```python
from build123d import *

# Parameters (mm, degrees)
SKETCH1_W           = 20
SKETCH1_H           = 16
BOSS_EXTRUDE1_DEPTH = 1.5
BOSS_EXTRUDE2_DEPTH = 2.6
CUT_EXTRUDE1_DEPTH  = 1
SKETCH4_R           = 1.85
CUT_EXTRUDE2_DEPTH  = 1.3
CUT_EXTRUDE3_DEPTH  = 4.3
FILLET1_R           = 1


with BuildPart() as part:
    # Sketch1 → Boss-Extrude1 (new body)
    with BuildSketch(Plane(origin=(0, 0, 0), x_dir=(1, 0, 0), z_dir=(0, 1, 0))):
        Rectangle(SKETCH1_W, SKETCH1_H)
    extrude(amount=BOSS_EXTRUDE1_DEPTH)

    # Sketch2 → Boss-Extrude2 (add)
    with BuildSketch(Plane.ZY.offset(10)):
        with BuildLine():
            Line((8, 0), (8, 5))
            Line((8, 5), (-5.076696831, 10))
            Line((-5.076696831, 10), (-13, 10))
            Line((-13, 10), (-13.5, 8.25))
            Line((-13.5, 8.25), (-16.8, 8.25))
            ThreePointArc((-16.8, 8.25), (-18.4, 5), (-16.8, 1.75))
            Line((-16.8, 1.75), (-13.5, 1.75))
            Line((-13.5, 1.75), (-13, 0))
            Line((-13, 0), (8, 0))
        make_face()
    boss_extrude2 = extrude(amount=-BOSS_EXTRUDE2_DEPTH)

    # Sketch3 → Cut-Extrude1 (cut)
    with BuildSketch(Plane(origin=(-7.4, 0, 0), x_dir=(0, 0, -1), z_dir=(1, 0, 0))):
        Polygon((-8, 1.5), (4.4, 1.5), (4.4, 9.7412585), (-8, 5), align=None)
    cut_extrude1 = extrude(amount=-CUT_EXTRUDE1_DEPTH, mode=Mode.SUBTRACT)

    # Sketch4 → Cut-Extrude2 (cut)
    with BuildSketch(Plane.ZY.offset(10)):
        Polygon((-18.672915143, 10), (-7, 10), (-7, 5), (-6.6, 0), (-8.743784953, 0), (-18.672915143, 0), align=None)
        with Locations((-13, 5)):
            Circle(SKETCH4_R, mode=Mode.SUBTRACT)
    cut_extrude2 = extrude(amount=-CUT_EXTRUDE2_DEPTH, mode=Mode.SUBTRACT)

    # Mirror1: Boss-Extrude2, Cut-Extrude1, Cut-Extrude2 across plane
    add(boss_extrude2.mirror(Plane(origin=(0, 0, 0), x_dir=(0, 0, 1), z_dir=(1, 0, 0))))
    add(cut_extrude1.mirror(Plane(origin=(0, 0, 0), x_dir=(0, 0, 1), z_dir=(1, 0, 0))), mode=Mode.SUBTRACT)
    add(cut_extrude2.mirror(Plane(origin=(0, 0, 0), x_dir=(0, 0, 1), z_dir=(1, 0, 0))), mode=Mode.SUBTRACT)

    # Sketch5 → Cut-Extrude3 (cut)
    with BuildSketch(Plane.XZ):
        with BuildLine():
            Line((-4.3, 6.2), (-3, 6.2))
            ThreePointArc((-3, 6.2), (-1, 4.2), (-3, 2.2))
            Line((-3, 2.2), (-4.3, 2.2))
            ThreePointArc((-4.3, 2.2), (-6.3, 4.2), (-4.3, 6.2))
        make_face()
        with BuildLine():
            Line((3, 6.2), (4.3, 6.2))
            ThreePointArc((4.3, 6.2), (6.3, 4.2), (4.3, 2.2))
            Line((4.3, 2.2), (3, 2.2))
            ThreePointArc((3, 2.2), (1, 4.2), (3, 6.2))
        make_face()
        with BuildLine():
            Line((-4.3, -1.6), (-3, -1.6))
            ThreePointArc((-3, -1.6), (-1, -3.6), (-3, -5.6))
            Line((-3, -5.6), (-4.3, -5.6))
            ThreePointArc((-4.3, -5.6), (-6.3, -3.6), (-4.3, -1.6))
        make_face()
        with BuildLine():
            Line((3, -1.6), (4.3, -1.6))
            ThreePointArc((4.3, -1.6), (6.3, -3.6), (4.3, -5.6))
            Line((4.3, -5.6), (3, -5.6))
            ThreePointArc((3, -5.6), (1, -3.6), (3, -1.6))
        make_face()
    extrude(amount=-CUT_EXTRUDE3_DEPTH, mode=Mode.SUBTRACT)

    # Fillet1
    fillet1_edges = [part.edges().sort_by_distance(p)[0] for p in [
        (-7.4, 5.62062925, -4.4),
        (10, 0, 0.7),
        (-10, 0, 0.7),
        (7.4, 5.62062925, -4.4),
    ]]
    fillet(fillet1_edges, radius=FILLET1_R - 0.0001)  # a hair under: the kernel refuses the full size


solid = part.part
```
For this review, take the finished solid that the model builds, in its own axes (mm). A direction names the side the tool comes from. Coordinates: 2 decimals unless noted, no trailing zeros. Order: outer loops, then holes, each group sorted by start corner. A loop starts at its lowest first (then second) coordinate and runs counter-clockwise, first axis right, second up. Notation, with made-up numbers: (-1.5, -7) - (44.5, -7) arc R18 cw to (44.5, 3) - close; hole circle Ø7 at (74.5, 64.25). An arc over 180 degrees is marked (long way). Answer as a JSON object with one key per item and string values. Group by question number.
1. For probe 1 along X at (y, z) = (2, -8.25); probe 2 along X at (y, z) = (7.5, -1.75); probe 3 along Y at (x, z) = (3.5, 6.25), list the stretches that pass through material, from the lowest coordinate up.
2. The part is to be moulded in two halves that separate along X. For faces 6 (the flat face through (-8.059, 9.137, -13.246)), 7 (the cylindrical face through (1, 0.7, -3.6)), 8 (the cylindrical face through (-9.699, 0.285, 0.763)), 9 (the flat face through (10, 5, -13)), say which applies: pulls with the +X half, pulls with the -X half, needs draft (parallel to the pull), parting line crosses it, or undercut.
3. Clearance check with flat-ended pins moving along their axes: P1, Ø5, axis at x = -1.5, z = -11.5, coming from the +Y side; P2, Ø1, axis at x = -8, z = -16, coming from the -Y side; P3, Ø1, axis at x = -0.5, z = -3.5, coming from the +Y side; P4, Ø1, axis at x = 8, z = -15, coming from the +Y side. State where each tip first meets the part, or that it passes through.
4. For faces 1 (the flat face through (0, 1, 8)), 2 (the flat face through (-8.059, 0.887, -13.254)), 3 (the cylindrical face through (-9.359, 5.556, -11.235)), 4 (the cylindrical face through (-1, 0.7, -3.6)), 5 (the flat face through (-8.4, 5, 1)), list the 3-axis set-ups (+Z, -Z, +X, -X, +Y, -Y) from which the entire face can be reached by the end or side of a thin tool; tool diameter is ignored.
5. We need section D-D on z = 4.2. State the section outline as (x, y) points, then the cut area to 3 significant figures.
6. We need section A-A on z = -12.25. State the section outline as (x, y) points, then the cut area to 3 significant figures.
7. We need section C-C on x = -1.75. State the section outline as (y, z) points.
Final values:
{
 "1": {"probe 1": "-8.7 to -7.4, 7.4 to 8.7", "probe 2": "-10 to -8.4, 8.4 to 10", "probe 3": "0 to 1.5"},
 "2": {"face 6": "needs draft", "face 7": "undercut", "face 8": "pulls with the -X half", "face 9": "pulls with the +X half"},
 "3": {"P1": "through", "P2": "y = 1.75", "P3": "y = 1.5", "P4": "y = 8.25"},
 "4": {"face 1": "+Z, +X, -X, +Y, -Y", "face 2": "-Z, +X, -X, -Y", "face 3": "-X", "face 4": "+Y, -Y", "face 5": "+Z, +Y"},
 "5": {"outline": "(-10, 1) arc R1 ccw to (-9, 0) - (-6.3, 0) - (-6.3, 1.5) - (-8.4, 1.5) - (-8.4, 6.45) - (-10, 6.45) - close; (-1, 0) - (1, 0) - (1, 1.5) - (-1, 1.5) - close; (6.3, 0) - (9, 0) arc R1 ccw to (10, 1) - (10, 6.45) - (8.4, 6.45) - (8.4, 1.5) - (6.3, 1.5) - close", "area": "29.5 mm²"},
 "6": {"outline": "(-10, 3.31) - (-8.7, 3.31) - (-8.7, 0) - (-7.4, 0) - (-7.4, 10) - (-8.7, 10) - (-8.7, 6.69) - (-10, 6.69) - close; (7.4, 0) - (8.7, 0) - (8.7, 3.31) - (10, 3.31) - (10, 6.69) - (8.7, 6.69) - (8.7, 10) - (7.4, 10) - close", "area": "34.8 mm²"},
 "7": {"outline": "(0, -8) - (1.5, -8) - (1.5, -5.16) - (0, -5.16) - close; (0, -2.04) - (1.5, -2.04) - (1.5, 2.64) - (0, 2.64) - close; (0, 5.76) - (1.5, 5.76) - (1.5, 8) - (0, 8) - close"}
}
